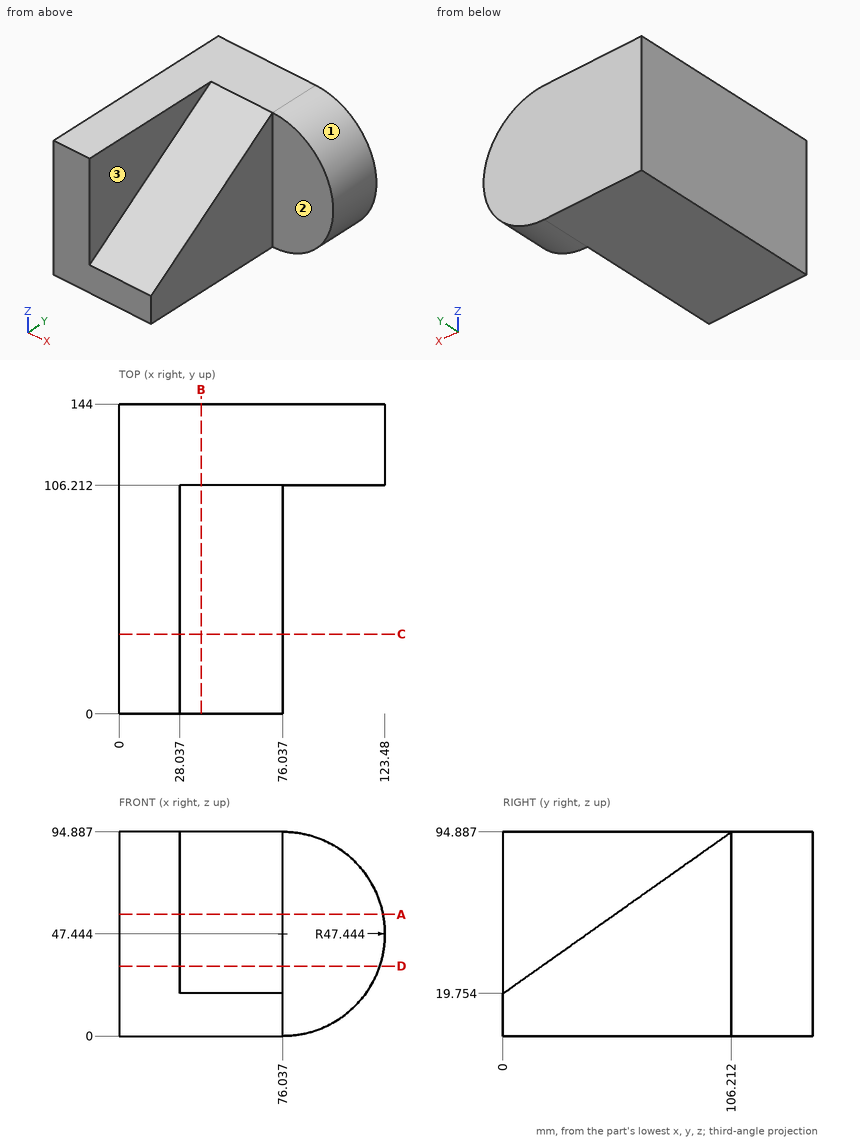
Verification items for this drawing (mm, ordinates from the low corner). A direction names the side the tool comes from. Coordinates: 2 decimals unless noted, no trailing zeros. Loops run counter-clockwise (first coordinate to the right, second up) from the corner with the lowest first, then second, coordinate; pieces in that order, holes last.
Item 1: Thickness scan on line 1 (X direction, y = 36.5, z = 79.5); line 2 (X direction, y = 91.5, z = 64); line 3 (Y direction, x = 81.5, z = 20). Record the ranges inside material, lowest first.
Item 2: Sectioned sample at C-C, the plane y = 37. Record the boundary of the cut face in (x, z), then the cut area to 4 significant figures.
Item 3: Go/stop test with flat-tipped pins: pin 1 Ø4 at (y, z) = (126, 41.5) entering from +X; pin 2 Ø3 at (x, z) = (52, 82.5) entering from -Y; pin 3 Ø4 at (x, z) = (67.5, 71.5) entering from -Y (1 decimal). Record where each tip stops, or that it passes through.
Item 4: Sectioned sample at A-A, the plane z = 56.5. Record the boundary of the cut face in (x, y), then the cut area to 3 significant figures.
Item 5: Access from +Z, -Z, +X, -X, +Y, -Y to the whole of each face (thin tool, end or side, straight path). Record for the marked faces 1, 2 and 3.
Item 6: Sectioned sample at B-B, the plane x = 38. Record the boundary of the cut face in (y, z).
Item 7: Sectioned sample at D-D, the plane z = 32.5. Record the boundary of the cut face in (x, y) (1 decimal), then the cut area to 3 significant figures.
Check result:
1. line 1: x = 0 to 28.04
1. line 2: x = 0 to 76.04
1. line 3: y = 106.21 to 144
2. outline: (0, 0) - (76.04, 0) - (76.04, 45.93) - (28.04, 45.93) - (28.04, 94.89) - (0, 94.89) - close
2. area: 4,865 mm2
3. pin 1: stops at x = 123.32
3. pin 2: stops at y = 86.58
3. pin 3: stops at y = 70.3
4. outline: (0, 0) - (28.04, 0) - (28.04, 51.95) - (76.04, 51.95) - (76.04, 106.21) - (122.61, 106.21) - (122.61, 144) - (0, 144) - close
4. area: 10,200 mm2
5. face 1: +X, +Y, -Y
5. face 2: +Z, -Z, +X, -Y
5. face 3: +Z, +X, -Y
6. outline: (0, 0) - (144, 0) - (144, 94.89) - (106.21, 94.89) - (0, 19.75) - close
7. outline: (0, 0) - (28, 0) - (28, 18) - (76, 18) - (76, 106.2) - (121.1, 106.2) - (121.1, 144) - (0, 144) - close
7. area: 11,800 mm2
